Build history of the part. All positions in model axes, mm. Give positions to 0.01 mm unless a question says otherwise; leave off trailing zeros. Write each loop counter-clockwise with the first axis right and the second up, starting at its lowest first coordinate (ties: lowest second). Pieces come first, ordered by that corner, then holes. Notation, with made-up numbers: (88, -24) -> (122, -24) arc R13 ccw to (122, -17) -> close; hole circle Ø5 at (4, 50). An arc over 180 degrees is marked (long way). One line per question, with ' | ' between items. Start each with the question number.
(1) Band-saw the part on B-B, the plane z = -107.5. Give the cut face in (x, y).
(2) Band-saw the part on C-C, the plane x = 2.6. Count the separate pieces of the cut face and the enclosed holes in it, and give its area (3 significant figures).
(3) Band-saw the part on A-A, the plane z = -355. Give the cut face in (x, y), and give its area (3 significant figures).
(4) Pin check, flat tips, straight feed: P1, Ø1.8, axis at x = 3.5, y = 3.5, coming from the -Z side; P2, Ø2, axis at x = 1.5, y = 129.5, coming from the -Z side; P3, Ø3, axis at x = 4, z = -2.5, coming from the +Y side. Stop position of each tip, or through.
(5) Drill centre lines: probe 1 along Y at (x, z) = (2.8, -421.5); probe 2 along Y at (x, z) = (4.15, -307.5); probe 3 along Y at (x, z) = (5.5, -191.5). Where is each one in solid material? Low to high. Write a range as from..to.
(6) Band-saw the part on D-D, the plane y = 199.5. Give the cut face in (x, z), and give its area (3 significant figures).
(7) Pull direction Y, two halves, no side cores. Call faces 1 (the flat face through (6, 99, -222)), 2 (the cylindrical face through (3.042, 213.594, -42.028)): released by +Y, released by -Y, zero draft, split by the parting line, or undercut.
from build123d import *

# Parameters (mm, degrees)
BOSS_EXTRUDE1_DEPTH = 6
SKETCH2_W           = 6
SKETCH2_H           = 37.5
CUT_EXTRUDE1_DEPTH  = 6
LPATTERN1_COUNT     = 4
LPATTERN1_PITCH     = 75
FILLET1_R           = 40
SKETCH3_W           = 6
SKETCH3_H           = 10
SKETCH3_H_2         = 112.5
CUT_EXTRUDE2_DEPTH  = 515.816472153
SKETCH4_W           = 15
SKETCH4_H           = 6
CUT_EXTRUDE3_DEPTH  = 515.816472153
SKETCH5_R           = 2
CUT_EXTRUDE4_DEPTH  = 515.816472153
SKETCH6_W           = 20
SKETCH6_H           = 6
CUT_EXTRUDE5_DEPTH  = 515.816472153
SKETCH7_R           = 2.5
CUT_EXTRUDE6_DEPTH  = 515.816472153


with BuildPart() as part:
    # Sketch1 → Boss-Extrude1 (new body)
    with BuildSketch(Plane(origin=(0, 0, 0), x_dir=(0, 0, -1), z_dir=(1, 0, 0))):
        Polygon((450, 225), (450, 250), (0, 250), (0, 0), (450, 0), (450, 127.5), (30, 127.5), (30, 225), align=None)
    extrude(amount=BOSS_EXTRUDE1_DEPTH)

    # Sketch2 → Cut-Extrude1 (cut)
    with BuildSketch(Plane(origin=(6, 0, 0), x_dir=(0, 0, -1), z_dir=(1, 0, 0))):
        with Locations((3, 231.25)):
            Rectangle(SKETCH2_W, SKETCH2_H)
    cut_extrude1 = extrude(amount=-CUT_EXTRUDE1_DEPTH, mode=Mode.SUBTRACT)

    # LPattern1: Cut-Extrude1 ×4
    with Locations(*[(0, -i * LPATTERN1_PITCH, 0) for i in range(1, LPATTERN1_COUNT)]):
        add(cut_extrude1, mode=Mode.SUBTRACT)

    # Fillet1
    fillet1_edges = [part.edges().sort_by_distance(p)[0] for p in [
        (3, 225, -30),
    ]]
    fillet(fillet1_edges, radius=FILLET1_R)

    # Sketch3 → Cut-Extrude2 (cut, through all)
    with BuildSketch(Plane.ZY):
        with Locations((-447, 230)):
            Rectangle(SKETCH3_W, SKETCH3_H)
        with Locations((-447, 56.25)):
            Rectangle(SKETCH3_W, SKETCH3_H_2)
    extrude(amount=-CUT_EXTRUDE2_DEPTH, mode=Mode.SUBTRACT)

    # Sketch4 → Cut-Extrude3 (cut, through all)
    with BuildSketch(Plane.ZY):
        with Locations((-23.5, 3)):
            Rectangle(SKETCH4_W, SKETCH4_H)
        with Locations((-426.5, 3)):
            Rectangle(SKETCH4_W, SKETCH4_H)
    extrude(amount=-CUT_EXTRUDE3_DEPTH, mode=Mode.SUBTRACT)

    # Sketch5 → Cut-Extrude4 (cut, through all)
    with BuildSketch(Plane.ZY):
        with Locations((-327.5, 243)):
            Circle(SKETCH5_R)
        with Locations((-307.5, 243)):
            Circle(SKETCH5_R)
        with BuildLine():
            Line((-362.5, 250), (-347.5, 250))
            ThreePointArc((-347.5, 250), (-355, 242.5), (-362.5, 250))
        make_face()
    extrude(amount=-CUT_EXTRUDE4_DEPTH, mode=Mode.SUBTRACT)

    # Sketch6 → Cut-Extrude5 (cut, through all)
    with BuildSketch(Plane.ZY):
        with Locations((-85, 3)):
            Rectangle(SKETCH6_W, SKETCH6_H)
    extrude(amount=-CUT_EXTRUDE5_DEPTH, mode=Mode.SUBTRACT)

    # Sketch7 → Cut-Extrude6 (cut, through all)
    with BuildSketch(Plane.ZY):
        with Locations((-421.5, 241.5)):
            Circle(SKETCH7_R)
        with Locations((-268.51, 241.5)):
            Circle(SKETCH7_R)
    extrude(amount=-CUT_EXTRUDE6_DEPTH, mode=Mode.SUBTRACT)


solid = part.part
Results:
1) outline: (0, 0) -> (6, 0) -> (6, 127.5) -> (0, 127.5) -> close; (0, 225) -> (6, 225) -> (6, 250) -> (0, 250) -> close
2) separate pieces: 1 | enclosed holes: 4 | area: 69,900 mm²
3) outline: (0, 0) -> (6, 0) -> (6, 127.5) -> (0, 127.5) -> close; (0, 225) -> (6, 225) -> (6, 242.5) -> (0, 242.5) -> close | area: 870 mm²
4) P1: stops at z = -444 | P2: stops at z = -30 | P3: stops at y = 212.5
5) probe 1: y = 6..127.5, 225..239, 244..250 | probe 2: y = 0..127.5, 225..241, 245..250 | probe 3: y = 0..127.5, 225..250
6) outline: (0, -32.72) -> (6, -32.72) -> (6, 0) -> (0, 0) -> close | area: 196 mm²
7) face 1: zero draft | face 2: undercut
